Study the drawing (mm; zero at the part's minimum x, y, z) and answer. A direction names the side the tool comes from. Round coordinates to 2 decimals unless told otherwise and drop trailing zeros. Order: outer loops, then holes, each group sorted by start corner. A loop starts at its lowest first (then second) coordinate and runs counter-clockwise, first axis right, second up. Notation, with made-up numbers: (87, 58) - (139, 58) arc R8 cw to (139, 70) - close; hole circle Ø3 at (-12, 71.5). An arc over 180 degrees is marked (long way). Use one line per item in the form item = value. Start each with the question number.
Q1. The part is cut by section D-D on x = 7.5. Determine the outline of the cut face in (y, z), plus the area to 3 significant figures.
Q2. The part is cut by section C-C on z = 8. Determine the outline of the cut face in (x, y), plus the area to 3 significant figures.
Q3. Which of the six approach directions +Z, -Z, +X, -X, +Y, -Y give full straight-line access (tool end or side, diameter ignored) to the marked faces 1, 2, 3 and 4?
Q4. The part is cut by section A-A on x = 15.75. Determine the outline of the cut face in (y, z).
Q5. The part is cut by section B-B on y = 13. Determine the outline of the cut face in (x, z), plus the area to 3 significant figures.
Q6. Find the intervals of material crossed by line 1 (X direction, y = 15.6, z = 3.9); line 2 (Y direction, x = 1.85, z = 3.5); line 3 (X direction, y = 14.5, z = 1), in increasing order. Write a range as [from, to].
Q7. Given P1, Ø1.5, axis at x = 2, y = 16, coming from the -Z side; P2, Ø3, axis at y = 14.5, z = 8.5, coming from the -X side; P3, Ø4, axis at y = 8.5, z = 10, coming from the +X side; P4, Ø3, axis at y = 9.5, z = 10, coming from the -X side, each flat-ended and moving along its own axis, determine where each tip first touches the part or whether it passes through.
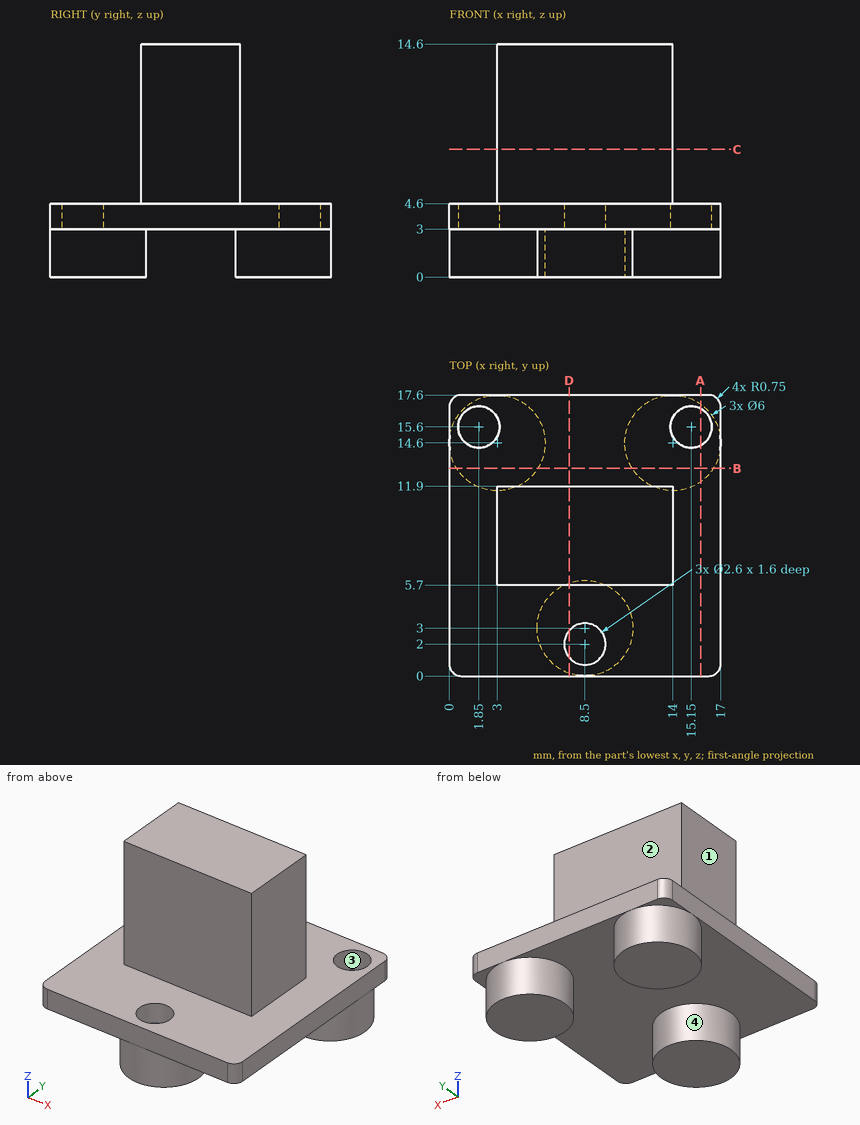
Found:
q1.outline = (0, 3) - (0.17, 3) - (0.17, 0) - (5.83, 0) - (5.83, 3) - (17.6, 3) - (17.6, 4.6) - (11.9, 4.6) - (11.9, 14.6) - (5.7, 14.6) - (5.7, 4.6) - (2.83, 4.6) - (2.83, 3) - (1.17, 3) - (1.17, 4.6) - (0, 4.6) - close
q1.area = 104 mm²
q2.outline = (3, 5.7) - (14, 5.7) - (14, 11.9) - (3, 11.9) - close
q2.area = 68.2 mm²
q3.face_1 = +Z, -X, +Y, -Y
q3.face_2 = +Z, +X, -X, +Y
q3.face_3 = +Z
q3.face_4 = -Z
q4.outline = (0, 3) - (12.16, 3) - (12.16, 0) - (17.04, 0) - (17.04, 3) - (17.6, 3) - (17.6, 4.6) - (16.75, 4.6) - (16.75, 3) - (14.45, 3) - (14.45, 4.6) - (0, 4.6) - close
q5.outline = (0, 3) - (0.46, 3) - (0.46, 0) - (5.54, 0) - (5.54, 3) - (11.46, 3) - (11.46, 0) - (16.54, 0) - (16.54, 3) - (17, 3) - (17, 4.6) - (0, 4.6) - close
q5.area = 57.7 mm²
q6.line_1 = [0, 0.55], [3.15, 13.85], [16.45, 17]
q6.line_2 = [0, 14.3], [16.9, 17.6]
q6.line_3 = [0, 6], [11, 17]
q7.P1 = 0
q7.P2 = through
q7.P3 = 14
q7.P4 = 3
